Build history of the part. All positions in model axes, mm. Face numbers are marked on the shaded views. A direction names the side the tool comes from. Coordinates: 2 decimals unless noted, no trailing zeros. Loops run counter-clockwise (first coordinate to the right, second up) from the corner with the lowest first, then second, coordinate; pieces in that order, holes last. Notation, with made-up numbers: (62.5, -39.75) - (121.5, -39.75) arc R16 ccw to (121.5, -30.75) - close; hole circle Ø9 at (58.25, 68.5). An arc over 180 degrees is marked (long way). One line per item, written item: value.
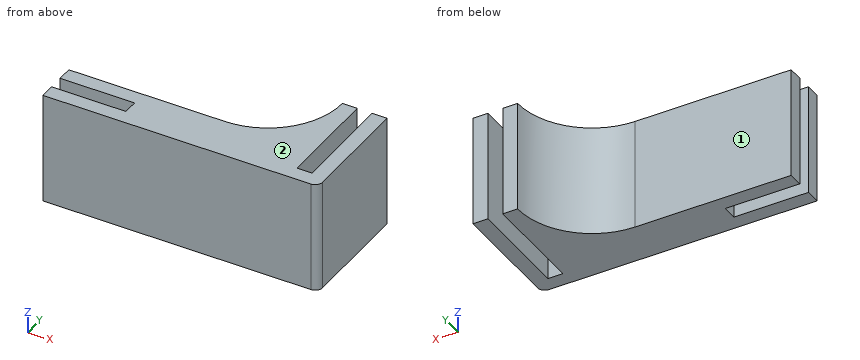
```python
from build123d import *

# Parameters (mm, degrees)
F1_DEPTH = 7.5
F2_R     = 9.99999
F3_R     = 1


# Not quite as in the source:
# - a fillet or chamfer is up to 0.001 mm smaller than in the source, because OpenCascade refuses the exact size


with BuildPart() as f1:
    # F0 (on Top) → F1 (new body, symmetric)
    with BuildSketch(Plane.XY):
        Polygon((-9.7452771891, 18.3048394923), (-9.7452771891, 8.3048394923), (-40.7452771891, 8.3048394923), (-40.7452771891, 6.3048394923), (-30.7452771891, 6.3048394923), (-30.7452771891, 4.3048394923), (-40.7452771891, 4.3048394923), (-40.7452771891, 2.3048394923), (-3.7452771891, 2.3048394923), (-3.7452771891, 18.3048394923), (-5.7452771891, 18.3048394923), (-5.7452771891, 4.3048394923), (-7.7452771891, 4.3048394923), (-7.7452771891, 18.3048394923), align=None)
    extrude(amount=F1_DEPTH, both=True)

    # F2 (radius 10 in the source; OpenCascade refuses exactly that, so slightly less here)
    f2_edges = [f1.edges().sort_by_distance(p)[0] for p in [
        (-9.745277, 8.304839, 0),
    ]]
    fillet(f2_edges, radius=F2_R)

    # F3
    f3_edges = [f1.edges().sort_by_distance(p)[0] for p in [
        (-3.745277, 2.304839, 0),
    ]]
    fillet(f3_edges, radius=F3_R)


solid = f1.part
```
Item 1: Cut at B-B, the plane y = 5.5. Write the cut outline in (x, z), then the cut area to 3 significant figures.
Check result:
outline: (-30.75, -7.5) - (-7.75, -7.5) - (-7.75, 7.5) - (-30.75, 7.5) - close; (-5.75, -7.5) - (-3.75, -7.5) - (-3.75, 7.5) - (-5.75, 7.5) - close
area: 375 mm^2
Item 2: Tool access for the marked faces 1 and 2: list every direction of +Z, -Z, +X, -X, +Y, -Y with a clear straight run to the whole face (end or side of a thin tool).
Check result:
face 1: +Z, -Z, -X, +Y
face 2: +Z, +X, -X, +Y, -Y
Item 3: Cut at D-D, the plane x = -24. Write the cut outline in (y, z).
Check result:
outline: (2.3, -7.5) - (8.3, -7.5) - (8.3, 7.5) - (2.3, 7.5) - close
Item 4: Probe probe 1 along X at (y, z) = (6.5, 4.5); probe 2 along Y at (x, z) = (-31.5, 4.75); probe 3 along X at (y, z) = (11.5, -6.5). List the from-to ranges inside material, lowest first. Write a range as from..to.
Check result:
probe 1: x = -40.75..-7.75, -5.75..-3.75
probe 2: y = 2.3..4.3, 6.3..8.3
probe 3: x = -12.42..-7.75, -5.75..-3.75
Item 5: Cut at A-A, the plane x = -36. Write the cut outline in (y, z).
Check result:
outline: (2.3, -7.5) - (4.3, -7.5) - (4.3, 7.5) - (2.3, 7.5) - close; (6.3, -7.5) - (8.3, -7.5) - (8.3, 7.5) - (6.3, 7.5) - close
Item 6: Drop flat-ended pins along their axis: P1, Ø8, axis at x = -37, z = -0.5, coming from the +Y side; P2, Ø7, axis at y = 13, z = 1.5, coming from the -X side; P3, Ø1, axis at x = -6.5, z = -3.5, coming from the +Y side. Give the stop position or say it passes through.
Check result:
P1: stops at y = 8.3
P2: stops at x = -15
P3: stops at y = 4.3
